from build123d import *

# Parameters (mm, degrees)
F0_R       = 27.7
F1_DEPTH   = 23.8
F2_SIZE2   = 11.9
F2_SIZE    = 2
F2_2_SIZE2 = 11.89999
F2_2_SIZE  = 1.99999


# Not quite as in the source:
# - a fillet or chamfer is up to 0.001 mm smaller than in the source, because OpenCascade refuses the exact size


with BuildPart() as f1:
    # F0 (on Front) → F1 (new body)
    with BuildSketch(Plane.XZ):
        with Locations((0.358, -0.004)):
            Circle(F0_R)
        Polygon((-2.222, -0.874), (-2.222, -0.004), (-2.222, 0.876), (-0.642, 0.876), (-0.642, 2.456), (1.108, 2.456), (1.108, 0.876), (2.688, 0.876), (2.688, -0.874), (1.108, -0.874), (1.108, -2.454), (-0.642, -2.454), (-0.642, -0.874), align=None, mode=Mode.SUBTRACT)
    extrude(amount=F1_DEPTH)

    # F2
    f2_edges = [f1.edges().sort_by_distance(p)[0] for p in [
        (-27.342, -23.8, -0.004),
    ]]
    f2_side = f1.faces().sort_by_distance((-26.558526, -23.8, -0.004))[0]
    chamfer(f2_edges, length=F2_SIZE, length2=F2_SIZE2, reference=f2_side)

    # F2#2 (size 2 and 11.9 in the source; OpenCascade refuses exactly that, so slightly less here)
    f2_2_edges = [f1.edges().sort_by_distance(p)[0] for p in [
        (-27.342, 0, -0.004),
    ]]
    f2_2_side = f1.faces().sort_by_distance((-26.558526, 0, -0.004))[0]
    chamfer(f2_2_edges, length=F2_2_SIZE, length2=F2_2_SIZE2, reference=f2_2_side)


solid = f1.part
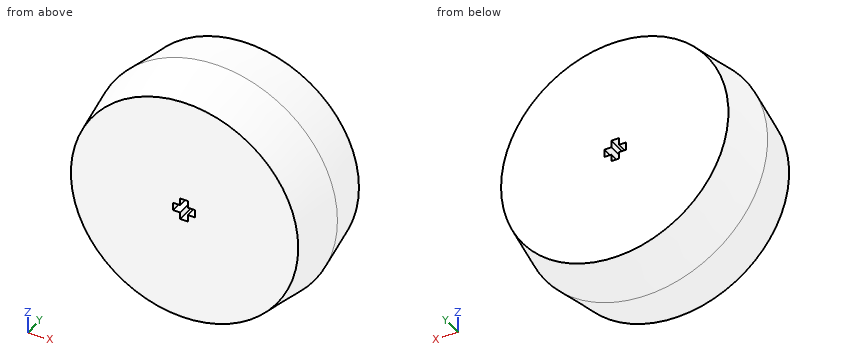
Read the model definition and answer for the solid it produces. Units are mm, in the model's axes. Round coordinates to 2 decimals unless told otherwise and drop trailing zeros. Loops run counter-clockwise (first coordinate to the right, second up) from the corner with the lowest first, then second, coordinate; pieces in that order, holes last. Notation, with made-up numbers: (18, 70.25) - (30, 70.25) arc R22 ccw to (30, 92.25) - close; hole circle Ø6 at (-21.5, 34.25). An arc over 180 degrees is marked (long way). One line per question, with ' | ' between items. Start each with the question number.
Q1. Section A-A on y = -2 is taken. Give the vertices of the cut face in (x, z).
Q2. Section B-B on y = -18.5 is taken. Give the vertices of the cut face in (x, z).
Q3. Find the intervals of material crossed by L1, parallel to X at y = -6.5, z = -7.5; L2, parallel to X at y = -3.5, z = 0; L3, parallel to Z at x = -3, y = -14.75, in increasing order.
Q4. Flat-ended cylindrical pins translate along their axes: pin 1 (0.8 mm diameter, centred on x = 2, y = -6.5, fed in from +Z); pin 2 (1.7 mm diameter, centred on y = -9.5, z = -1.5, fed in from +X); pin 3 (10 mm diameter, centred on x = -3.5, y = -17.5, fed in from +Z). Find the tip coordinate at first contact, or state that the pin passes through.
Established:
1) outline: circle Ø52.07 at (0.36, 0); hole (-2.22, -0.87) - (-0.64, -0.87) - (-0.64, -2.45) - (1.11, -2.45) - (1.11, -0.87) - (2.69, -0.87) - (2.69, 0.88) - (1.11, 0.88) - (1.11, 2.46) - (-0.64, 2.46) - (-0.64, 0.88) - (-2.22, 0.88) - close
2) outline: circle Ø53.18 at (0.36, 0); hole (-2.22, -0.87) - (-0.64, -0.87) - (-0.64, -2.45) - (1.11, -2.45) - (1.11, -0.87) - (2.69, -0.87) - (2.69, 0.88) - (1.11, 0.88) - (1.11, 2.46) - (-0.64, 2.46) - (-0.64, 0.88) - (-2.22, 0.88) - close
3) L1: -25.36 to 26.08 | L2: -25.93 to -2.22, 2.69 to 26.65 | L3: -27.02 to 27.01
4) pin 1: z = 26.81 | pin 2: x = 27.76 | pin 3: z = 27.46
